Design review of the part built by this model. Coordinates are the model's own, in mm. Coordinates: 2 decimals unless noted, no trailing zeros. Answer as a JSON object with one key per item and string values. Group by question number.
1. Consider section A-A (z = 2.5). Count the separate pieces of the cut face and the enclosed holes in it, then the cut area to 3 significant figures.
2. To check wall thickness, follow probe 1 along X at (y, z) = (64.5, 1.1); probe 2 along X at (y, z) = (83.5, 1.75); probe 3 along X at (y, z) = (66, 1.1). State the ranges of each line that lie inside material, in increasing order.
3. Insertion check: pin 1 (1.6 mm diameter, centred on x = 52, z = 1, fed in from -Y); pin 2 (1 mm diameter, centred on y = 74, z = 0.5, fed in from -X). Each pin has a flat end and moves straight along its axis. Give the tip position at first contact, or say it passes through.
from build123d import *

# Parameters (mm, degrees)
BASE_DEPTH           = 3.175
SKETCH3_R            = 4.7625
SKETCH3_R_2          = 1.25
FASTENERS_DEPTH      = 4.175
FILLET1_R            = 10
TOPOLOGY_HOLES_DEPTH = 4.175
SKETCH6_R            = 1.25
SUPPORTS_DEPTH       = 4.175
SKETCH8_R            = 11.5
SKETCH8_R_2          = 1.25
MOTOR_PLATE_DEPTH    = 4.175
SKETCH12_R           = 1.25
PLATE_SUPPORT_DEPTH  = 3.175


with BuildPart() as part:
    # Base Sketch → Base (new body)
    with BuildSketch(Plane.XY):
        Polygon((0, 0), (-17.207293091, 24.574561329), (103.396353455, 109.022143775), (224, 24.574561329), (206.792706909, 0), (103.396353455, 72.398906112), align=None)
    extrude(amount=BASE_DEPTH)

    # Sketch3 → Fasteners (cut, through all)
    with BuildSketch(Plane.XY.offset(3.175)):
        with Locations((103.396353455, 90.710524944)):
            Circle(SKETCH3_R)
        with Locations((103.396353455, 81.198024944)):
            Circle(SKETCH3_R_2)
        with Locations((111.634420108, 95.466774944)):
            Circle(SKETCH3_R_2)
        with Locations((95.158286801, 95.466774944)):
            Circle(SKETCH3_R_2)
    extrude(amount=-FASTENERS_DEPTH, mode=Mode.SUBTRACT)

    # Fillet1
    fillet1_edges = [part.edges().sort_by_distance(p)[0] for p in [
        (103.396353455, 109.022143775, 1.5875),
        (103.396353455, 72.398906112, 1.5875),
    ]]
    fillet(fillet1_edges, radius=FILLET1_R)

    # Sketch5 → Topology Holes (cut, through all)
    with BuildSketch(Plane.XY.offset(3.175)):
        with BuildLine():
            Line((45.265276935, 43.461284839), (46.55138053, 46.994825426))
            ThreePointArc((46.55138053, 46.994825426), (47.649729084, 48.426221129), (49.370458393, 48.968764996))
            Line((49.370458393, 48.968764996), (53.130773743, 48.968764996))
            ThreePointArc((53.130773743, 48.968764996), (55.038207644, 47.570176595), (54.277926615, 45.330460907))
            Line((54.277926615, 45.330460907), (48.29181505, 41.138940464))
            ThreePointArc((48.29181505, 41.138940464), (45.927139319, 41.190537872), (45.265276935, 43.461284839))
        make_face()
        with BuildLine():
            Line((33.938973564, 34.656761682), (29.055875209, 34.656761682))
            ThreePointArc((29.055875209, 34.656761682), (25.779267032, 36.362455937), (25.297104726, 40.024842255))
            Line((25.297104726, 40.024842255), (26.967222725, 44.613453746))
            ThreePointArc((26.967222725, 44.613453746), (28.431687463, 46.52198135), (30.725993208, 47.245373173))
            Line((30.725993208, 47.245373173), (35.609091563, 47.245373173))
            ThreePointArc((35.609091563, 47.245373173), (38.88569974, 45.539678918), (39.367862046, 41.8772926))
            Line((39.367862046, 41.8772926), (37.697744047, 37.288681109))
            ThreePointArc((37.697744047, 37.288681109), (36.233279309, 35.380153505), (33.938973564, 34.656761682))
        make_face()
        with BuildLine():
            Line((45.69398528, 54.219312743), (46.980088875, 57.752853329))
            ThreePointArc((46.980088875, 57.752853329), (46.318226492, 60.023600296), (43.953550761, 60.075197704))
            Line((43.953550761, 60.075197704), (37.967439195, 55.883677261))
            ThreePointArc((37.967439195, 55.883677261), (37.207158167, 53.643961574), (39.114592068, 52.245373173))
            Line((39.114592068, 52.245373173), (42.874907418, 52.245373173))
            ThreePointArc((42.874907418, 52.245373173), (44.595636727, 52.78791704), (45.69398528, 54.219312743))
        make_face()
        with BuildLine():
            Line((84.750405047, 73.654491311), (89.633503402, 73.654491311))
            ThreePointArc((89.633503402, 73.654491311), (91.927809147, 74.377883134), (93.392273885, 76.286410738))
            Line((93.392273885, 76.286410738), (95.062391884, 80.875022229))
            ThreePointArc((95.062391884, 80.875022229), (94.580229578, 84.537408548), (91.303621401, 86.243102802))
            Line((91.303621401, 86.243102802), (86.420523046, 86.243102802))
            ThreePointArc((86.420523046, 86.243102802), (84.1262173, 85.519710979), (82.661752563, 83.611183375))
            Line((82.661752563, 83.611183375), (80.991634563, 79.022571885))
            ThreePointArc((80.991634563, 79.022571885), (81.473796869, 75.360185566), (84.750405047, 73.654491311))
        make_face()
        with BuildLine():
            Line((75.094219674, 77.438579645), (73.808116079, 73.905039059))
            ThreePointArc((73.808116079, 73.905039059), (72.709767526, 72.473643356), (70.989038217, 71.931099489))
            Line((70.989038217, 71.931099489), (67.228722867, 71.931099489))
            ThreePointArc((67.228722867, 71.931099489), (65.321288966, 73.32968789), (66.081569994, 75.569403577))
            Line((66.081569994, 75.569403577), (72.06768156, 79.76092402))
            ThreePointArc((72.06768156, 79.76092402), (74.432357291, 79.709326612), (75.094219674, 77.438579645))
        make_face()
        with BuildLine():
            Line((74.665511329, 66.680551741), (73.379407734, 63.147011155))
            ThreePointArc((73.379407734, 63.147011155), (74.041270118, 60.876264188), (76.405945849, 60.82466678))
            Line((76.405945849, 60.82466678), (82.392057414, 65.016187223))
            ThreePointArc((82.392057414, 65.016187223), (83.152338443, 67.25590291), (81.244904542, 68.654491311))
            Line((81.244904542, 68.654491311), (77.484589192, 68.654491311))
            ThreePointArc((77.484589192, 68.654491311), (75.763859883, 68.111947444), (74.665511329, 66.680551741))
        make_face()
    topology_holes = extrude(amount=-TOPOLOGY_HOLES_DEPTH, mode=Mode.SUBTRACT)

    # Sketch6 → Supports (cut, through all)
    with BuildSketch(Plane.XY.offset(3.175)):
        with Locations((69.888485086, 54.429929741)):
            Circle(SKETCH6_R)
        with Locations((62.516116687, 49.267741813)):
            Circle(SKETCH6_R)
        with Locations((50.471011524, 66.469934744)):
            Circle(SKETCH6_R)
        with Locations((57.843379923, 71.632122671)):
            Circle(SKETCH6_R)
        with Locations((148.949326987, 71.632122671)):
            Circle(SKETCH6_R)
        with Locations((156.321695386, 66.469934744)):
            Circle(SKETCH6_R)
        with Locations((144.276590222, 49.267741813)):
            Circle(SKETCH6_R)
        with Locations((136.904221824, 54.429929741)):
            Circle(SKETCH6_R)
    extrude(amount=-SUPPORTS_DEPTH, mode=Mode.SUBTRACT)

    # Mirror1: Topology Holes across plane
    add(topology_holes.mirror(Plane(origin=(103.396353455, 0, 0), x_dir=(0, 0, 1), z_dir=(1, 0, 0))), mode=Mode.SUBTRACT)

    # Sketch8 → Motor Plate (cut, through all)
    with BuildSketch(Plane.XY.offset(3.175)):
        with Locations((5.321938208, 22.038080082)):
            Circle(SKETCH8_R)
        with Locations((-8.465370335, 24.46915457)):
            Circle(SKETCH8_R_2)
        with Locations((7.753012695, 35.825388624)):
            Circle(SKETCH8_R_2)
        with Locations((19.10924675, 19.607005595)):
            Circle(SKETCH8_R_2)
        with Locations((2.89086372, 8.25077154)):
            Circle(SKETCH8_R_2)
        with Locations((203.901843189, 8.25077154)):
            Circle(SKETCH8_R_2)
        with Locations((215.258077244, 24.46915457)):
            Circle(SKETCH8_R_2)
        with Locations((199.039694214, 35.825388624)):
            Circle(SKETCH8_R_2)
        with Locations((187.68346016, 19.607005595)):
            Circle(SKETCH8_R_2)
        with Locations((201.470768702, 22.038080082)):
            Circle(SKETCH8_R)
    extrude(amount=-MOTOR_PLATE_DEPTH, mode=Mode.SUBTRACT)

    # Sketch12 → Plate Support (add)
    with BuildSketch(Plane.XY.offset(3.175)):
        Polygon((-3.441458618, 4.914912266), (-10.593055004, -0.092689434), (-20.917430859, 14.652047363), (-13.765834472, 19.659649063), align=None)
        with Locations((-10.573341227, 5.414599951)):
            Circle(SKETCH12_R, mode=Mode.SUBTRACT)
        with Locations((-15.735529154, 12.786968349)):
            Circle(SKETCH12_R, mode=Mode.SUBTRACT)
        Polygon((210.234165528, 4.914912266), (217.385761914, -0.092689434), (227.710137768, 14.652047363), (220.558541382, 19.659649063), align=None)
        with Locations((217.366048137, 5.414599951)):
            Circle(SKETCH12_R, mode=Mode.SUBTRACT)
        with Locations((222.528236064, 12.786968349)):
            Circle(SKETCH12_R, mode=Mode.SUBTRACT)
    extrude(amount=-PLATE_SUPPORT_DEPTH)


solid = part.part
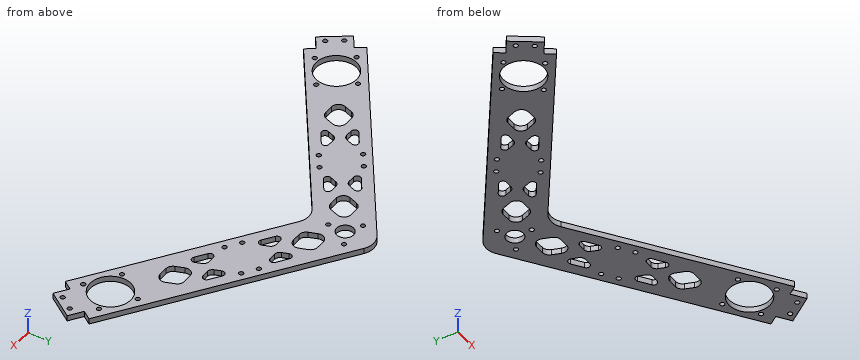
Findings below:
{
 "1": {"separate pieces": "1", "enclosed holes": "38", "area": "6,470 mm^2"},
 "2": {"probe 1": "x = 39.81 to 73.87, 81.65 to 92.12, 114.68 to 125.14, 132.92 to 166.98", "probe 2": "x = 66.95 to 82.62, 95.1 to 111.69, 124.17 to 139.85", "probe 3": "x = 41.95 to 49.31, 51.63 to 74.42, 83.13 to 94.26, 112.53 to 123.66, 132.37 to 155.16, 157.48 to 164.84"},
 "3": {"pin 1": "stops at y = 35.85", "pin 2": "stops at x = 52.67"}
}
